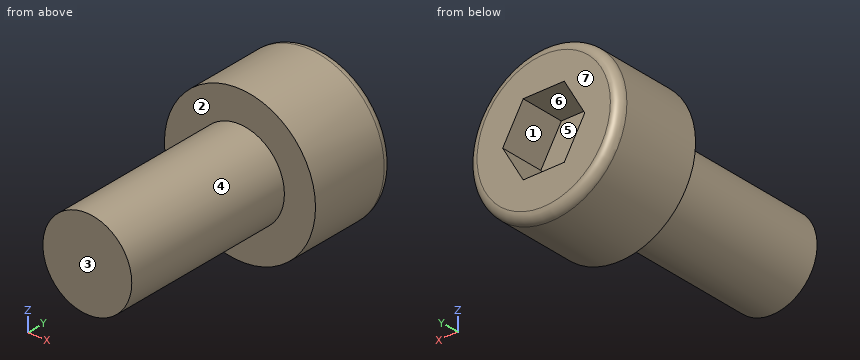
Autodesk Inventor part; units mm, degrees
ref_plane "YZ Plane" through (0, 0, 0) normal (1, 0, 0) x (0, 1, 0)
ref_plane "XZ Plane" through (0, 0, 0) normal (0, 1, 0) x (-1, 0, 0)
ref_plane "XY Plane" through (0, 0, 0) normal (0, 0, 1) x (1, 0, 0)
sketch "Cap Cross Section" plane through (0, 0, 0) normal (0, 1, 0) x (-1, 0, 0)
  circle A0 centre (0, 0) radius 4.25
  dimension "d0" = 8.5
extrude "Cap" add sketch "Cap Cross Section" along normal blind 5
sketch "Key Socket Cutout Outline" plane through (0, 5, 0) normal (0, 1, 0) x (1, 0, 0)
  line L0 (1.1547, 2) -> (2.3094, 0)
  line L1 (2.3094, 0) -> (1.1547, -2)
  line L2 (1.1547, -2) -> (-1.1547, -2)
  line L3 (-1.1547, -2) -> (-2.3094, 0)
  line L4 (-2.3094, 0) -> (-1.1547, 2)
  line L5 (-1.1547, 2) -> (1.1547, 2)
  point P0 (0, 0)
  point P1 (0, 0)
  dimension "d3" = 4
extrude "Key Socket Cutout" cut sketch "Key Socket Cutout Outline" against normal blind 2.5
sketch "Body Cross Section" plane through (0, 0, 0) normal (0, -1, 0) x (1, 0, 0)
  circle A0 centre (0, 0) radius 2.5
  dimension "d6" = 5
extrude "Body" add sketch "Body Cross Section" along normal blind 10
thread "Thread"
fillet "Cap Fillet" radius 0.5 1 edges at (4.25, 5, 0)
properties part number "SSCF-M5-10-A4" material "Stainless Steel AISI 317"
Geometry check sheet. Reference: the model listing, model coordinates, mm. Face numbers are marked on the shaded views. A direction names the side the tool comes from. Round coordinates to 2 decimals unless told otherwise and drop trailing zeros. Loops run counter-clockwise (first coordinate to the right, second up) from the corner with the lowest first, then second, coordinate; pieces in that order, holes last. Notation, with made-up numbers: (-39.75, 79.5) - (-20.75, 79.5) arc R10 ccw to (-20.75, 95.5) - close; hole circle Ø8 at (-20.75, 74.5). An arc over 180 degrees is marked (long way). Write each question's results on one line, items separated by ' | '. Start each with the question number.
Q1. Thickness scan on line 1 (Y direction, x = 0.25, z = -1); line 2 (Y direction, x = 3, z = 1); line 3 (X direction, y = -9, z = -1.5). Record the ranges inside material, lowest first. Write a range as [from, to].
Q2. Cross-section at C-C on y = 0.5. Enter the section's corners in (x, z).
Q3. Cross-section at A-A on y = 3.75. Enter the section's corners in (x, z), and give its area (3 significant figures).
Q4. Access from +Z, -Z, +X, -X, +Y, -Y to the whole of each face (thin tool, end or side, straight path). Record for the marked faces 1, 2 and 3.
Q5. Cross-section at B-B on x = 0. Enter the section's corners in (y, z), and give its area (3 significant figures).
Q6. Cross-section at D-D on y = -2. Enter the section's corners in (x, z), and give its area (3 significant figures).
Q7. Release check for a two-part mould opening along Z. For the marked faces 4, 5, 6 and 7 record: +Z half, -Z half, draft (parallel to the pull), parting line (faces both ways), or undercut.
Q8. Gauge pin test, flat ends, axial feed: P1, Ø1.5, axis at y = -6, z = -1.5, coming from the -X side; P2, Ø3, axis at x = 0.5, z = -1, coming from the +Y side; P3, Ø3, axis at y = -3, z = 0.5, coming from the +X side. Record the tip position at first contact, or that the pin passes through.
Answers below:
1) line 1: y = [-10, 2.5] | line 2: y = [0, 5] | line 3: x = [-2, 2]
2) outline: circle Ø8.5 at (0, 0)
3) outline: circle Ø8.5 at (0, 0); hole (-2.31, 0) - (-1.15, -2) - (1.15, -2) - (2.31, 0) - (1.15, 2) - (-1.15, 2) - close | area: 42.9 mm²
4) face 1: +Y | face 2: -Y | face 3: +Z, -Z, +X, -X, -Y
5) outline: (-10, -2.5) - (0, -2.5) - (0, -4.25) - (4.5, -4.25) arc R0.5 ccw to (5, -3.75) - (5, -2) - (2.5, -2) - (2.5, 2) - (5, 2) - (5, 3.75) arc R0.5 ccw to (4.5, 4.25) - (0, 4.25) - (0, 2.5) - (-10, 2.5) - close | area: 82.4 mm²
6) outline: circle Ø5 at (0, 0) | area: 19.6 mm²
7) face 4: parting line | face 5: undercut | face 6: undercut | face 7: draft
8) P1: stops at x = -2.38 | P2: stops at y = 5 | P3: stops at x = 2.5
